Here's the drawing with two shaded views (mm, measured from the low corner). I have some questions. A direction names the side the tool comes from. Give positions to 0.01 mm unless a question says otherwise; leave off trailing zeros. Loops run counter-clockwise (first coordinate to the right, second up) from the corner with the lowest first, then second, coordinate; pieces in that order, holes last. Notation, with made-up numbers: (83.5, 63) - (127.5, 63) arc R21 cw to (127.5, 96) - close; hole circle Ø11 at (48.5, 70). An arc over 180 degrees is marked (long way). Answer as a JSON object with one key per item and string values. Group by question number.
Item 1: Suppose I cut it at D-D on z = 19.25. Write out the boundary of the cut face in (x, y).
Item 2: Which directions (+Z, -Z, +X, -X, +Y, -Y) give clear straight access to the entire face, cutting with the end or side of a thin tool? Please do the marked faces 1, 2 and 3.
Item 3: Suppose I cut it at A-A on y = 4.75. Write out the boundary of the cut face in (x, z), and give its area (3 significant figures).
Item 4: Will these pins go through, and if not, where does the flat tip stop? pin 1 (1.5 mm diameter, centred on x = 7, z = 19, fed in from +Y); pin 2 (0.8 mm diameter, centred on x = 0.5, z = 15, fed in from +Y).
Item 5: Please list where these lines run through material, in increasing order: L1, parallel to Z at x = 31, y = 6.5; L2, parallel to X at y = 3.75, z = 12; L3, parallel to X at y = 4.5, z = 26.5.
Item 6: Thinking about a two-plate mould opening in Z: for the marked faces 4, 5 and 6, which applies, pulls with the +Z half, pulls with the -Z half, needs draft (parallel to the pull), parting line crosses it, or undercut?
Item 7: Suppose I cut it at B-B on x = 32. Write out the boundary of the cut face in (y, z).
Item 8: Suppose I cut it at C-C on z = 14.5. Write out the boundary of the cut face in (x, y), and give its area (3 significant figures).
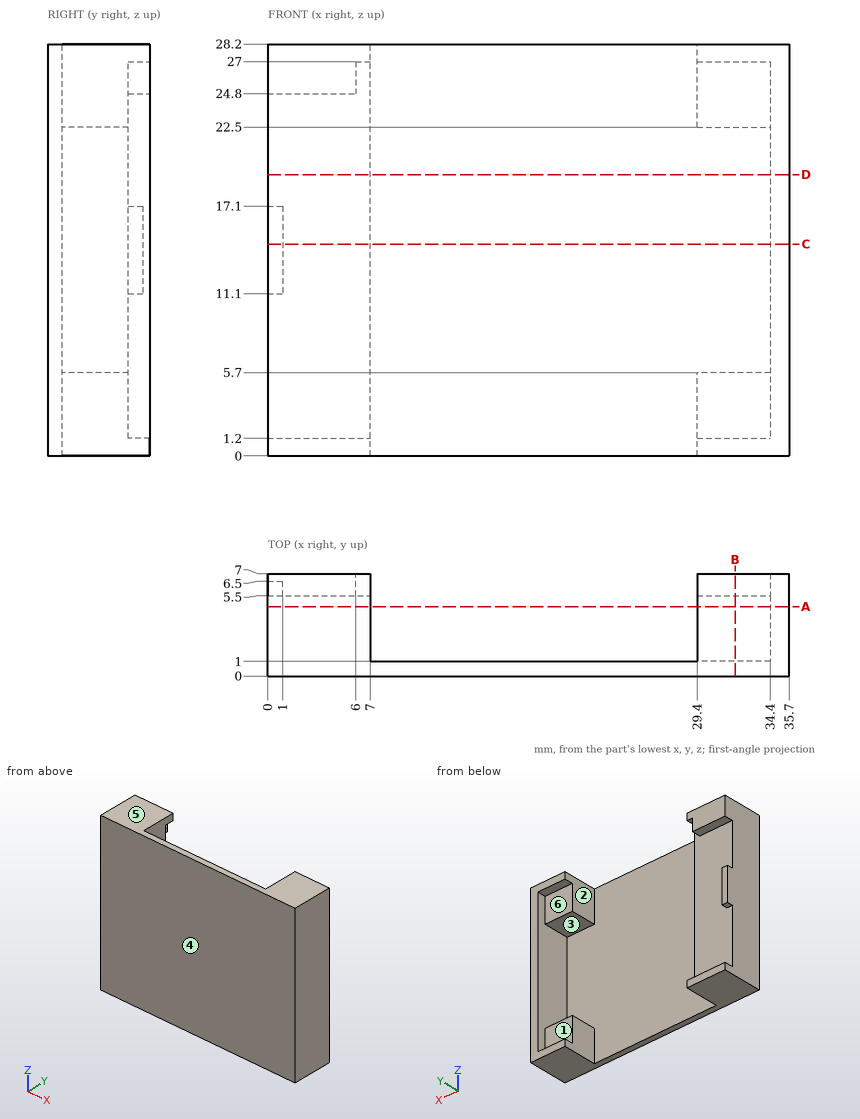
Worked out:
{
 "1": {"outline": "(0, 0) - (35.7, 0) - (35.7, 7) - (34.4, 7) - (34.4, 1) - (7, 1) - (7, 5.5) - (0, 5.5) - close"},
 "2": {"face 1": "-X, +Y", "face 2": "+Z, -Z, +Y", "face 3": "+Y"},
 "3": {"outline": "(0, 0) - (7, 0) - (7, 28.2) - (0, 28.2) - close; (29.4, 0) - (35.7, 0) - (35.7, 28.2) - (29.4, 28.2) - (29.4, 22.5) - (34.4, 22.5) - (34.4, 5.7) - (29.4, 5.7) - close", "area": "291 mm2"},
 "4": {"pin 1": "stops at y = 5.5", "pin 2": "stops at y = 6.5"},
 "5": {"L1": "z = 0 to 1.2, 27 to 28.2", "L2": "x = 0 to 7, 34.4 to 35.7", "L3": "x = 0 to 7, 29.4 to 35.7"},
 "6": {"face 4": "needs draft", "face 5": "pulls with the +Z half", "face 6": "undercut"},
 "7": {"outline": "(0, 0) - (7, 0) - (7, 1.2) - (5.5, 1.2) - (5.5, 5.7) - (1, 5.7) - (1, 22.5) - (5.5, 22.5) - (5.5, 27) - (7, 27) - (7, 28.2) - (0, 28.2) - close"},
 "8": {"outline": "(0, 0) - (35.7, 0) - (35.7, 7) - (34.4, 7) - (34.4, 1) - (7, 1) - (7, 5.5) - (1, 5.5) - (1, 6.5) - (0, 6.5) - close", "area": "76.0 mm2"}
}
